The model under review builds one solid part; all positions refer to its coordinate system, in mm. Face numbers are marked on the shaded views. A direction names the side the tool comes from. Round coordinates to 2 decimals unless told otherwise and drop trailing zeros. Order: outer loops, then holes, each group sorted by start corner. A loop starts at its lowest first (then second) coordinate and runs counter-clockwise, first axis right, second up. Notation, with made-up numbers: (-17.75, 32.5) -> (21.25, 32.5) arc R16 cw to (21.25, 49.5) -> close; hole circle Ø9 at (34.25, 54.25). An arc over 180 degrees is marked (long way). Use a Markdown table: item, result. Add a question column.
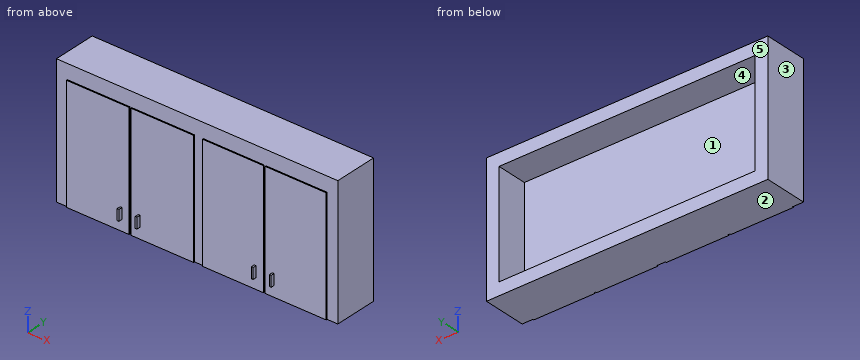
```python
from build123d import *

# Parameters (mm, degrees)
F0_W     = 1981.2
F0_H     = 914.4
F1_DEPTH = 304.8
F2_W     = 441.96
F2_H     = 810.768
F2_W_2   = 429.26
F3_DEPTH = 7.62
F4_W     = 12.7
F4_H     = 76.2
F5_DEPTH = 25.4
F6_W     = 1803.4
F6_H     = 736.6
F7_DEPTH = 215.9


with BuildPart() as f1:
    # F0 (on Front) → F1 (new body)
    with BuildSketch(Plane.XZ):
        with Locations((990.6, 457.2)):
            Rectangle(F0_W, F0_H)
    extrude(amount=-F1_DEPTH)

    # F2 (on face) → F3 (join)
    with BuildSketch(Plane.XZ):
        with Locations((297.18, 405.384)):
            Rectangle(F2_W, F2_H)
        with Locations((751.84, 405.384)):
            Rectangle(F2_W, F2_H)
        with Locations((1248.41, 405.384)):
            Rectangle(F2_W_2, F2_H)
        with Locations((1690.37, 405.384)):
            Rectangle(F2_W_2, F2_H)
    extrude(amount=F3_DEPTH)

    # F4 (on face) → F5 (join)
    with BuildSketch(Plane.XZ.offset(7.62)):
        with Locations((1532.89, 114.3)):
            Rectangle(F4_W, F4_H)
        with Locations((1405.89, 114.3)):
            Rectangle(F4_W, F4_H)
        with Locations((588.01, 114.3)):
            Rectangle(F4_W, F4_H)
        with Locations((461.01, 114.3)):
            Rectangle(F4_W, F4_H)
    extrude(amount=F5_DEPTH)

    # F6 (on face) → F7 (cut)
    with BuildSketch(Plane(origin=(0, 304.8, 0), x_dir=(-1, 0, 0), z_dir=(0, 1, 0))):
        with Locations((-990.6, 457.2)):
            Rectangle(F6_W, F6_H)
    extrude(amount=-F7_DEPTH, mode=Mode.SUBTRACT)


solid = f1.part
```
Q1. Wall thickness on line 1 (Z direction, x = 1119, y = 148.5); line 2 (X direction, y = 266.5, z = 691.5); line 3 (Z direction, x = 1819.5, y = -2): over which ranges is each line inside the solid? List them lowest first. Write a range as [from, to].
Q2. Add section B-B (z = 583). Write out the cut boundary in (x, y), then the cut area to 3 significant figures.
Q3. Add section C-C (y = 245). Write out the cut boundary in (x, z), then the cut area to 3 significant figures.
Q4. Machinability: for the marked faces 4 and 5, which of the approach directions +Z, -Z, +X, -X, +Y, -Y give a long, thin tool a straight path to every point of the face, cutting with its end or side? Answer none if there is none.
Q5. Add section A-A (x = 1211). Write out the cut boundary in (y, z), then the cut area to 3 significant figures.
Q6. Insertion check: pin 1 (5 mm diameter, centred on x = 262.5, y = 22, fed in from -Z); pin 2 (7.5 mm diameter, centred on y = -17.5, z = 100.5, fed in from +X); pin 3 (14 mm diameter, centred on x = 1404.5, y = -24.5, fed in from +Z); pin 4 (8.5 mm diameter, centred on y = -4.5, z = 353.5, fed in from +X). Each pin has a flat end and moves straight along its axis. Give the tip position at first contact, or say it passes through.
Q7. Mouldability with a two-part tool opening along X and no side actions: class the marked faces 1, 2 and 3 as pulls with the +X half, pulls with the -X half, needs draft (parallel to the pull), parting line crosses it, or undercut.
Report:
| question | item | result |
|---|---|---|
| 1 | line 1 | z = [0, 88.9], [825.5, 914.4] |
| 1 | line 2 | x = [0, 88.9], [1892.3, 1981.2] |
| 1 | line 3 | z = [0, 810.77] |
| 2 | outline | (0, 0) -> (76.2, 0) -> (76.2, -7.62) -> (518.16, -7.62) -> (518.16, 0) -> (530.86, 0) -> (530.86, -7.62) -> (972.82, -7.62) -> (972.82, 0) -> (1033.78, 0) -> (1033.78, -7.62) -> (1463.04, -7.62) -> (1463.04, 0) -> (1475.74, 0) -> (1475.74, -7.62) -> (1905, -7.62) -> (1905, 0) -> (1981.2, 0) -> (1981.2, 304.8) -> (1892.3, 304.8) -> (1892.3, 88.9) -> (88.9, 88.9) -> (88.9, 304.8) -> (0, 304.8) -> close |
| 2 | area | 228,000 mm² |
| 3 | outline | (0, 0) -> (1981.2, 0) -> (1981.2, 914.4) -> (0, 914.4) -> close; hole (88.9, 88.9) -> (1892.3, 88.9) -> (1892.3, 825.5) -> (88.9, 825.5) -> close |
| 3 | area | 483,000 mm² |
| 4 | face 4 | +Y |
| 4 | face 5 | +Z, -Z, +X, -X, +Y |
| 5 | outline | (-7.62, 0) -> (304.8, 0) -> (304.8, 88.9) -> (88.9, 88.9) -> (88.9, 825.5) -> (304.8, 825.5) -> (304.8, 914.4) -> (0, 914.4) -> (0, 810.77) -> (-7.62, 810.77) -> close |
| 5 | area | 126,000 mm² |
| 6 | pin 1 | stops at z = 0 |
| 6 | pin 2 | stops at x = 1539.24 |
| 6 | pin 3 | stops at z = 152.4 |
| 6 | pin 4 | stops at x = 1905 |
| 7 | face 1 | undercut |
| 7 | face 2 | needs draft |
| 7 | face 3 | pulls with the -X half |
